```python
from build123d import *

# Parameters (mm, degrees)
F3_01_CONTINUOUSSOCKETBODY_D9_70_DEPTH     = 9.7
SKETCH_2_W                                 = 30.8
SKETCH_2_H                                 = 12.55
F3_02_FLANGEBLANK_TOZ4_70_DEPTH            = 4.7
SKETCH_3_R                                 = 2.5
F3_03_FIXEDPOSTBLANK_TOZ8_20_DEPTH         = 8.2
SKETCH_4_W                                 = 30.8
SKETCH_4_H                                 = 12.55
F3_04_FRONTRELIEF_TOZ4_10_DEPTH            = 4.1
F3_05_RESTOREPROTRUDINGSOCKETNOSE_DEPTH    = 4.2
F3_06_DRECEIVEROUTERPOCKET_D4_10_DEPTH     = 4.1
F3_07_DRECEIVERINNERISLAND_DEPTH           = 4.2
SKETCH_8_R                                 = 0.575
F3_08_9CONTACTHOLES_DIA1_15_D4_50_DEPTH    = 4.5
SKETCH_9_R                                 = 0.675
F3_09_EQUIVALENTLEADIN_DIA1_35_D0_25_DEPTH = 0.25
SKETCH_10_R                                = 1.6
F3_10_FIXEDPOSTBORES_DIA3_20_DEPTH         = 8.3


with BuildPart() as part:
    # 草图1 → F3_01_ContinuousSocketBody_D9.70 (new body)
    with BuildSketch(Plane.XY):
        with BuildLine():
            Line((-9.063773303, 4.75), (9.063773303, 4.75))
            ThreePointArc((9.063773303, 4.75), (9.671973947, 4.469703739), (9.853983675, 3.825229941))
            Line((9.853983675, 3.825229941), (8.606615254, -4.074770059))
            ThreePointArc((8.606615254, -4.074770059), (8.336108621, -4.558200644), (7.816404882, -4.75))
            Line((7.816404882, -4.75), (-7.816404882, -4.75))
            ThreePointArc((-7.816404882, -4.75), (-8.336108621, -4.558200644), (-8.606615254, -4.074770059))
            Line((-8.606615254, -4.074770059), (-9.853983675, 3.825229941))
            ThreePointArc((-9.853983675, 3.825229941), (-9.671973947, 4.469703739), (-9.063773303, 4.75))
        make_face()
    extrude(amount=F3_01_CONTINUOUSSOCKETBODY_D9_70_DEPTH)

    # 草图2 → F3_02_FlangeBlank_ToZ4.70 (add)
    with BuildSketch(Plane.XY):
        Rectangle(SKETCH_2_W, SKETCH_2_H)
    extrude(amount=F3_02_FLANGEBLANK_TOZ4_70_DEPTH)

    # 草图3 → F3_03_FixedPostBlank_ToZ8.20 (add)
    with BuildSketch(Plane.XY):
        with Locations(Location((-12.5, 0, 0), (0, 0, 180))):
            Circle(SKETCH_3_R)
        with Locations(Location((12.5, 0, 0), (0, 0, 180))):
            Circle(SKETCH_3_R)
    extrude(amount=F3_03_FIXEDPOSTBLANK_TOZ8_20_DEPTH)

    # 草图4 → F3_04_FrontRelief_ToZ4.10 (cut)
    with BuildSketch(Plane.XY):
        Rectangle(SKETCH_4_W, SKETCH_4_H)
    extrude(amount=F3_04_FRONTRELIEF_TOZ4_10_DEPTH, mode=Mode.SUBTRACT)

    # 草图5 → F3_05_RestoreProtrudingSocketNose (add)
    with BuildSketch(Plane.XY):
        with BuildLine():
            Line((-9.063773303, 4.75), (9.063773303, 4.75))
            ThreePointArc((9.063773303, 4.75), (9.671973947, 4.469703739), (9.853983675, 3.825229941))
            Line((9.853983675, 3.825229941), (8.606615254, -4.074770059))
            ThreePointArc((8.606615254, -4.074770059), (8.336108621, -4.558200644), (7.816404882, -4.75))
            Line((7.816404882, -4.75), (-7.816404882, -4.75))
            ThreePointArc((-7.816404882, -4.75), (-8.336108621, -4.558200644), (-8.606615254, -4.074770059))
            Line((-8.606615254, -4.074770059), (-9.853983675, 3.825229941))
            ThreePointArc((-9.853983675, 3.825229941), (-9.671973947, 4.469703739), (-9.063773303, 4.75))
        make_face()
    extrude(amount=F3_05_RESTOREPROTRUDINGSOCKETNOSE_DEPTH)

    # 草图6 → F3_06_DReceiverOuterPocket_D4.10 (cut)
    with BuildSketch(Plane.XY):
        with BuildLine():
            Line((-7.444046944, 4.3), (7.444046944, 4.3))
            ThreePointArc((7.444046944, 4.3), (8.154188345, 3.952900706), (8.316575127, 3.179331535))
            Line((8.316575127, 3.179331535), (6.596807685, -3.620668465))
            ThreePointArc((6.596807685, -3.620668465), (6.277180209, -4.110141401), (5.724279503, -4.3))
            Line((5.724279503, -4.3), (-5.724279503, -4.3))
            ThreePointArc((-5.724279503, -4.3), (-6.277180209, -4.110141401), (-6.596807685, -3.620668465))
            Line((-6.596807685, -3.620668465), (-8.316575127, 3.179331535))
            ThreePointArc((-8.316575127, 3.179331535), (-8.154188345, 3.952900706), (-7.444046944, 4.3))
        make_face()
    extrude(amount=F3_06_DRECEIVEROUTERPOCKET_D4_10_DEPTH, mode=Mode.SUBTRACT)

    # 草图7 → F3_07_DReceiverInnerIsland (add)
    with BuildSketch(Plane.XY):
        with BuildLine():
            Line((-7.047021477, 3.3), (7.047021477, 3.3))
            ThreePointArc((7.047021477, 3.3), (7.371118761, 3.13443752), (7.426924294, 2.774804754))
            Line((7.426924294, 2.774804754), (5.515560657, -3.025195246))
            ThreePointArc((5.515560657, -3.025195246), (5.37009536, -3.224097284), (5.135657841, -3.3))
            Line((5.135657841, -3.3), (-5.135657841, -3.3))
            ThreePointArc((-5.135657841, -3.3), (-5.37009536, -3.224097284), (-5.515560657, -3.025195246))
            Line((-5.515560657, -3.025195246), (-7.426924294, 2.774804754))
            ThreePointArc((-7.426924294, 2.774804754), (-7.371118761, 3.13443752), (-7.047021477, 3.3))
        make_face()
    extrude(amount=F3_07_DRECEIVERINNERISLAND_DEPTH)

    # 草图8 → F3_08_9ContactHoles_Dia1.15_D4.50 (cut)
    with BuildSketch(Plane.XY):
        with Locations((-5.54, 1.42)):
            Circle(SKETCH_8_R)
        with Locations((-2.77, 1.42)):
            Circle(SKETCH_8_R)
        with Locations((0, 1.42)):
            Circle(SKETCH_8_R)
        with Locations((2.77, 1.42)):
            Circle(SKETCH_8_R)
        with Locations((5.54, 1.42)):
            Circle(SKETCH_8_R)
        with Locations((-4.155, -1.42)):
            Circle(SKETCH_8_R)
        with Locations((-1.385, -1.42)):
            Circle(SKETCH_8_R)
        with Locations((1.385, -1.42)):
            Circle(SKETCH_8_R)
        with Locations((4.155, -1.42)):
            Circle(SKETCH_8_R)
    extrude(amount=F3_08_9CONTACTHOLES_DIA1_15_D4_50_DEPTH, mode=Mode.SUBTRACT)

    # 草图9 → F3_09_EquivalentLeadIn_Dia1.35_D0.25 (cut)
    with BuildSketch(Plane.XY):
        with Locations((-5.54, 1.42)):
            Circle(SKETCH_9_R)
        with Locations((-2.77, 1.42)):
            Circle(SKETCH_9_R)
        with Locations((0, 1.42)):
            Circle(SKETCH_9_R)
        with Locations((2.77, 1.42)):
            Circle(SKETCH_9_R)
        with Locations((5.54, 1.42)):
            Circle(SKETCH_9_R)
        with Locations((-4.155, -1.42)):
            Circle(SKETCH_9_R)
        with Locations((-1.385, -1.42)):
            Circle(SKETCH_9_R)
        with Locations((1.385, -1.42)):
            Circle(SKETCH_9_R)
        with Locations((4.155, -1.42)):
            Circle(SKETCH_9_R)
    extrude(amount=F3_09_EQUIVALENTLEADIN_DIA1_35_D0_25_DEPTH, mode=Mode.SUBTRACT)

    # 草图10 → F3_10_FixedPostBores_Dia3.20 (cut)
    with BuildSketch(Plane.XY):
        with Locations(Location((-12.5, 0, 0), (0, 0, 180))):
            Circle(SKETCH_10_R)
        with Locations(Location((12.5, 0, 0), (0, 0, 180))):
            Circle(SKETCH_10_R)
    extrude(amount=F3_10_FIXEDPOSTBORES_DIA3_20_DEPTH, mode=Mode.SUBTRACT)


solid = part.part
```
The model under review builds one solid part; all positions refer to its coordinate system, in mm. A direction names the side the tool comes from. Coordinates: 2 decimals unless noted, no trailing zeros. Write each loop counter-clockwise with the first axis right and the second up, starting at its lowest first coordinate (ties: lowest second). Pieces come first, ordered by that corner, then holes. Notation, with made-up numbers: (55.25, 62.25) -> (83.25, 62.25) arc R33 cw to (83.25, 98.25) -> close; hole circle Ø8 at (-4, 80.5). An arc over 180 degrees is marked (long way). One line per item, written item: value. Start each with the question number.
Q1. To check wall thickness, follow probe 1 along Y at (x, z) = (2.77, 1.4) (3 decimals); probe 2 along X at (y, z) = (-2, 7.25); probe 3 along X at (y, z) = (0.75, 5). State the ranges of each line that lie inside material, in increasing order.
Q2. Add section B-B, the plane x = 12.5. Give the boundary of the cut face in (y, z) (3 decimals), then the cut area to 3 significant figures.
Q3. The part is to be moulded in two halves that separate along Y. For faces 3 (the face through (-4.2, -1.4, 4.5)), 4 (the face through (-0.7, -4.6, 0)), 5 (the face through (-5.5, 1.4, 4.5)), 6 (the face through (0, 4.75, 7)), say which applies: +Y half, -Y half, draft (parallel to the pull), parting line (faces both ways), or undercut.
Q4. Add section A-A, the plane z = 7. Give the boundary of the cut face in (x, y), then the cut area to 3 significant figures.
Q5. Add section C-C, the plane z = 1.25. Count the separate pieces of the cut face and the enclosed holes in it, then the cut area to 3 significant figures.
Q6. For faces 1 (the face through (0, -4.75, 7)), 2 (the face through (1.916, -1.64, 2.345)), list the 3-axis set-ups (+Z, -Z, +X, -X, +Y, -Y) from which the entire face can be reached by the end or side of a thin tool; tool diameter is ignored.
Q7. Clearance check with flat-ended pins moving along their axes: P1, Ø0.7, axis at x = -4, y = -1.5, coming from the -Z side; P2, Ø4, axis at y = 2.5, z = 1.5, coming from the -X side; P3, Ø2, axis at x = -1.5, z = 2.5, coming from the +Y side. State where each tip first meets the part, or that it passes through.
Q8. Add section D-D, the plane x = 0. Give the boundary of the cut face in (y, z) (3 decimals), then the cut area to 3 significant figures.
Response:
1. probe 1: -4.75 to -4.3, -3.3 to 0.845, 1.995 to 3.3, 4.3 to 4.75
1. probe 2: -14 to -11, -8.93 to 8.93, 11 to 14
1. probe 3: -14.88 to -13.91, -11.09 to -10.12, -9.37 to 9.37, 10.12 to 11.09, 13.91 to 14.88
2. outline: (-6.275, 4.1) -> (-1.6, 4.1) -> (-1.6, 8.2) -> (-2.5, 8.2) -> (-2.5, 4.7) -> (-6.275, 4.7) -> close; (1.6, 4.1) -> (6.275, 4.1) -> (6.275, 4.7) -> (2.5, 4.7) -> (2.5, 8.2) -> (1.6, 8.2) -> close
2. area: 11.9 mm²
3. face 3: undercut
3. face 4: draft
3. face 5: undercut
3. face 6: +Y half
4. outline: circle Ø5 at (-12.5, 0); (-9.85, 3.83) -> (-8.61, -4.07) arc R0.8 ccw to (-7.82, -4.75) -> (7.82, -4.75) arc R0.8 ccw to (8.61, -4.07) -> (9.85, 3.83) arc R0.8 ccw to (9.06, 4.75) -> (-9.06, 4.75) arc R0.8 ccw to start; circle Ø5 at (12.5, 0); hole circle Ø3.2 at (-12.5, 0); hole circle Ø3.2 at (12.5, 0)
4. area: 198 mm²
5. separate pieces: 2
5. enclosed holes: 10
5. area: 123 mm²
6. face 1: +Z, +X, -X, -Y
6. face 2: -Z
7. P1: z = 4.5
7. P2: x = -9.86
7. P3: y = 4.75
8. outline: (-6.275, 4.1) -> (-4.75, 4.1) -> (-4.75, 0) -> (-4.3, 0) -> (-4.3, 4.1) -> (-3.3, 4.1) -> (-3.3, 0) -> (0.745, 0) -> (0.745, 0.25) -> (0.845, 0.25) -> (0.845, 4.5) -> (1.995, 4.5) -> (1.995, 0.25) -> (2.095, 0.25) -> (2.095, 0) -> (3.3, 0) -> (3.3, 4.1) -> (4.3, 4.1) -> (4.3, 0) -> (4.75, 0) -> (4.75, 4.1) -> (6.275, 4.1) -> (6.275, 4.7) -> (4.75, 4.7) -> (4.75, 9.7) -> (-4.75, 9.7) -> (-4.75, 4.7) -> (-6.275, 4.7) -> close
8. area: 80.6 mm²
